Verification items for the finished model (mm, model axes). Face numbers are marked on the shaded views. A direction names the side the tool comes from. Give positions to 0.01 mm unless a question says otherwise; leave off trailing zeros. Write each loop counter-clockwise with the first axis right and the second up, starting at its lowest first coordinate (ties: lowest second). Pieces come first, ordered by that corner, then holes. Notation, with made-up numbers: (7, -39) - (35, -39) arc R20 ccw to (35, -9) - close; hole circle Ø6 at (1.5, -27). An arc over 180 degrees is marked (long way). Put each result on its own line as item: value.
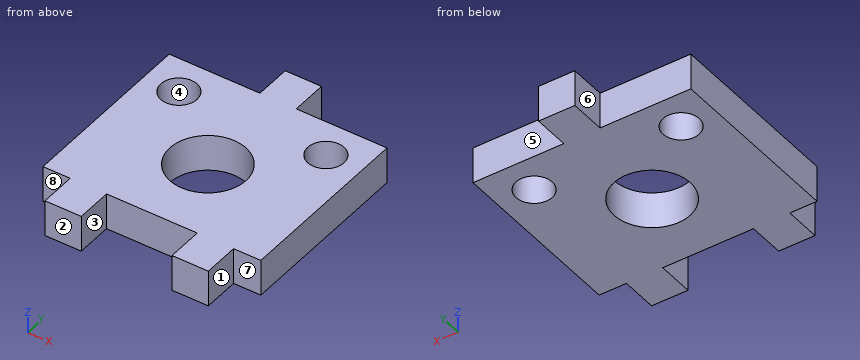
Autodesk Inventor part; units mm, degrees
ref_plane "YZ Plane" through (0, 0, 0) normal (1, 0, 0) x (0, 1, 0)
ref_plane "XZ Plane" through (0, 0, 0) normal (0, 1, 0) x (-1, 0, 0)
ref_plane "XY Plane" through (0, 0, 0) normal (0, 0, 1) x (1, 0, 0)
sketch "Sketch1" plane through (0, 0, 0) normal (0, 0, 1) x (1, 0, 0)
  circle A0 centre (44.45, 27.9405) radius 6.985 construction
  circle A1 centre (18.5683, 50.8) radius 6.35 construction
  line L0 (6.35, 63.5) -> (6.35, 50.8) construction
  line L1 (6.35, 50.8) -> (19.05, 50.8) construction
  line L2 (19.05, 50.8) -> (19.05, 63.5) construction
  line L3 (19.05, 63.5) -> (6.35, 63.5) construction
  circle A2 centre (70.0106, 50.8) radius 6.35 construction
  line L4 (31.779, 27.94) -> (38.1948, 39.0525) construction
  line L5 (38.1948, 39.0525) -> (51.0264, 39.0525) construction
  line L6 (51.0264, 39.0525) -> (57.4422, 27.94) construction
  line L7 (57.4422, 27.94) -> (51.0264, 16.8275) construction
  line L8 (51.0264, 16.8275) -> (38.1948, 16.8275) construction
  line L9 (6.35, 63.5) -> (6.35, 0)
  line L10 (82.55, 0) -> (82.55, 63.5)
  line L11 (82.55, 63.5) -> (6.35, 63.5)
  line L12 (31.779, 27.94) -> (38.1948, 16.8275) construction
  line L13 (44.45, 0) -> (44.45, 27.9405) construction
  line L14 (44.45, 27.9405) -> (44.45, 63.5) construction
  line L15 (44.45, 0) -> (60.325, 0)
  line L16 (44.45, 0) -> (60.325, 0)
  line L17 (73.025, 0) -> (73.025, -12.7)
  line L18 (73.025, -12.7) -> (60.325, -12.7)
  line L19 (60.325, -12.7) -> (60.325, 0)
  line L20 (73.025, 0) -> (82.55, 0)
  line L21 (44.45, 0) -> (28.575, 0)
  line L22 (44.45, 0) -> (28.575, 0)
  line L23 (15.875, 0) -> (15.875, -12.7)
  line L24 (15.875, -12.7) -> (28.575, -12.7)
  line L25 (28.575, -12.7) -> (28.575, 0)
  line L26 (15.875, 0) -> (6.35, 0)
  point P0 (0, 0)
  point P1 (0, 0)
  point P2 (12.8606, 0)
  dimension "d0" = 76.2
  dimension "d1" = 63.5
  dimension "d21" = 15.875
  dimension "d22" = 0
  dimension "d24" = 12.7
  dimension "d25" = 12.7
extrude "Extrusion1" add sketch "Sketch1" along normal blind 12.7
sketch "Sketch2" plane through (0, 0, 12.7) normal (0, 0, 1) x (1, 0, 0)
  circle A0 centre (18.5683, 50.8) radius 6.35
  line L0 (31.779, 27.94) -> (38.1948, 39.0525) construction
  line L1 (44.45, 0) -> (44.45, 15.875) construction
  line L2 (38.1948, 39.0525) -> (51.0264, 39.0525) construction
  line L3 (51.0264, 16.8275) -> (38.1948, 16.8275) construction
  circle A1 centre (44.6106, 27.94) radius 13.335
  line L4 (51.0264, 39.0525) -> (57.4422, 27.94) construction
  line L5 (57.4422, 27.94) -> (51.0264, 16.8275) construction
  circle A2 centre (70.0106, 50.8) radius 6.35
  line L6 (44.45, 0) -> (44.45, 27.94) construction
  line L7 (31.779, 27.94) -> (38.1948, 16.8275) construction
  line L8 (44.45, 0) -> (44.45, 27.94) construction
  line L9 (6.35, 63.5) -> (82.55, 63.5) construction
  line L10 (44.45, 27.94) -> (44.45, 63.5) construction
  line L11 (82.55, 63.5) -> (6.35, 63.5) construction
  dimension "d8" = 26.67
  dimension "d9" = 12.7
  dimension "d10" = 12.7
  dimension "d17" = 27.94
extrude "Extrusion2" cut sketch "Sketch2" against normal blind 12.7
sketch "Sketch3" plane through (0, 0, 12.7) normal (0, 0, 1) x (1, 0, 0)
  line L0 (28.575, 0) -> (60.325, 0) construction
  line L1 (44.45, 0) -> (44.45, 63.5) construction
  line L2 (82.55, 63.5) -> (6.35, 63.5) construction
  line L3 (44.45, 63.5) -> (44.45, 69.85) construction
  line L4 (38.1, 76.2) -> (50.8, 76.2)
  line L5 (50.8, 76.2) -> (50.8, 63.5)
  line L6 (50.8, 63.5) -> (38.1, 63.5)
  line L7 (38.1, 63.5) -> (38.1, 76.2)
  line L8 (38.1, 76.2) -> (50.8, 63.5) construction
  line L9 (50.8, 76.2) -> (38.1, 63.5) construction
  point P0 (0, 0)
  dimension "d26" = 6.35
  dimension "d27" = 12.7
  dimension "d28" = 12.7
extrude "Extrusion3" add sketch "Sketch3" against normal blind 12.7
properties part number "Near Holder" material "PVC-Piping"
Q1. Scan lines: line 1 along X through (y, z) = (-7.5, 1) (3 decimals); line 2 along X through (y, z) = (55, 12); line 3 along Y through (x, z) = (67, 10). Record each from-to range of solid material in increasing order.
Answers follow:
line 1: x = 15.875 to 28.575, 60.325 to 73.025
line 2: x = 6.35 to 13.81, 23.33 to 65.25, 74.77 to 82.55
line 3: y = -12.7 to 45.21, 56.39 to 63.5
Q2. Section check A-A, the plane y = 50.8. Record the cut outline in (x, z).
Answers follow:
outline: (6.35, 0) - (12.22, 0) - (12.22, 12.7) - (6.35, 12.7) - close; (24.92, 0) - (63.66, 0) - (63.66, 12.7) - (24.92, 12.7) - close; (76.36, 0) - (82.55, 0) - (82.55, 12.7) - (76.36, 12.7) - close
Q3. Section check B-B, the plane y = 27.94. Record the cut outline in (x, z).
Answers follow:
outline: (6.35, 0) - (31.28, 0) - (31.28, 12.7) - (6.35, 12.7) - close; (57.95, 0) - (82.55, 0) - (82.55, 12.7) - (57.95, 12.7) - close
Q4. Go/stop test with flat-tipped pins: pin 1 Ø6.5 at (y, z) = (-5, 8) entering from -X (3 decimals); pin 2 Ø3 at (x, z) = (79, 9) entering from -Y; pin 3 Ø5 at (x, z) = (19.5, 7) entering from +Y. Record where each tip stops, or that it passes through.
Answers follow:
pin 1: stops at x = 15.875
pin 2: stops at y = 0
pin 3: stops at y = 63.5
Q5. Set-up check for the marked faces 5, 6, 7 and 8: record each of +Z, -Z, +X, -X, +Y, -Y from which the full face is reachable in a straight line by a thin tool's end or side.
Answers follow:
face 5: +Z, -Z, +X, +Y
face 6: +Z, -Z, -X, +Y
face 7: +Z, -Z, +X, -Y
face 8: +Z, -Z, -X, -Y
Q6. Section check C-C, the plane z = 11. Record the cut outline in (x, y) (3 decimals).
Answers follow:
outline: (6.35, 0) - (15.875, 0) - (15.875, -12.7) - (28.575, -12.7) - (28.575, 0) - (60.325, 0) - (60.325, -12.7) - (73.025, -12.7) - (73.025, 0) - (82.55, 0) - (82.55, 63.5) - (50.8, 63.5) - (50.8, 76.2) - (38.1, 76.2) - (38.1, 63.5) - (6.35, 63.5) - close; hole circle Ø12.7 at (18.568, 50.8); hole circle Ø26.67 at (44.611, 27.94); hole circle Ø12.7 at (70.011, 50.8)
Q7. Section check D-D, the plane x = 74. Record the cut outline in (y, z).
Answers follow:
outline: (0, 0) - (45.86, 0) - (45.86, 12.7) - (0, 12.7) - close; (55.74, 0) - (63.5, 0) - (63.5, 12.7) - (55.74, 12.7) - close
Q8. Release check for a two-part mould opening along X. For the marked faces 1, 2, 3 and 4 record: released by +X, released by -X, zero draft, split by the parting line, or undercut.
Answers follow:
face 1: released by +X
face 2: zero draft
face 3: undercut
face 4: undercut
